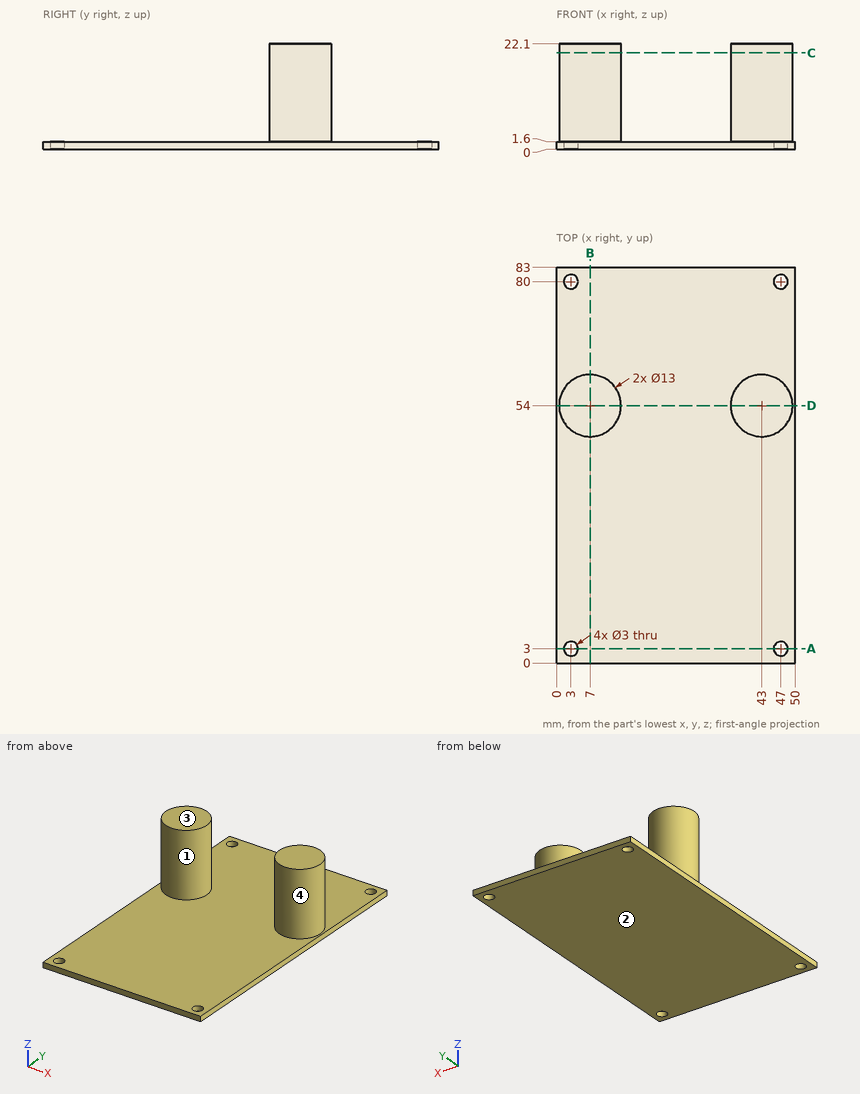
Design review of the part shown in the three views and the two pictorial views. Dimensions are in mm from the part's minimum x, y and z. A direction names the side the tool comes from. Round coordinates to 2 decimals unless told otherwise and drop trailing zeros. Loops run counter-clockwise (first coordinate to the right, second up) from the corner with the lowest first, then second, coordinate; pieces in that order, holes last.
1) Tool access review of the marked faces 3 and 4: name each direction out of +Z, -Z, +X, -X, +Y, -Y from which nothing blocks a thin tool from reaching the whole face with its end or side.
Values follow:
face 3: +Z, +X, -X, +Y, -Y
face 4: +Z
2) Clearance check with flat-ended pins moving along their axes: P1, Ø6, axis at y = 46, z = 8.5, coming from the +X side; P2, Ø8, axis at x = 29.5, y = 23.5, coming from the +Z side; P3, Ø1.8, axis at x = 3, y = 3, coming from the +Z side; P4, Ø8, axis at x = 35.5, z = 10, coming from the -Y side. State where each tip first meets the part, or that it passes through.
Values follow:
P1: stops at x = 47.15
P2: stops at z = 1.6
P3: passes through
P4: stops at y = 48.52
3) Consider section D-D on y = 54. State the section outline as (x, z) points, then the cut area to 3 significant figures.
Values follow:
outline: (0, 0) - (50, 0) - (50, 1.6) - (49.5, 1.6) - (49.5, 22.1) - (36.5, 22.1) - (36.5, 1.6) - (13.5, 1.6) - (13.5, 22.1) - (0.5, 22.1) - (0.5, 1.6) - (0, 1.6) - close
area: 613 mm2
4) Consider section B-B on x = 7. State the section outline as (y, z) points, then the cut area to 3 significant figures.
Values follow:
outline: (0, 0) - (83, 0) - (83, 1.6) - (60.5, 1.6) - (60.5, 22.1) - (47.5, 22.1) - (47.5, 1.6) - (0, 1.6) - close
area: 399 mm2
5) Wall thickness on line 1 along Y through (x, z) = (3, 0.4); line 2 along X through (y, z) = (80, 0.8); line 3 along Z through (x, y) = (14.5, 55.5): over which ranges is each line inside the solid? List them lowest first.
Values follow:
line 1: y = 0 to 1.5, 4.5 to 78.5, 81.5 to 83
line 2: x = 0 to 1.5, 4.5 to 45.5, 48.5 to 50
line 3: z = 0 to 1.6
6) Consider section A-A on y = 3. State the section outline as (x, z) points, then the cut area to 3 significant figures.
Values follow:
outline: (0, 0) - (1.5, 0) - (1.5, 1.6) - (0, 1.6) - close; (4.5, 0) - (45.5, 0) - (45.5, 1.6) - (4.5, 1.6) - close; (48.5, 0) - (50, 0) - (50, 1.6) - (48.5, 1.6) - close
area: 70.4 mm2
7) The part is to be moulded in two halves that separate along X. For the marked faces 1 and 2, say which applies: pulls with the +X half, pulls with the -X half, needs draft (parallel to the pull), parting line crosses it, or undercut.
Values follow:
face 1: undercut
face 2: needs draft
8) Consider section C-C on z = 20.25. State the section outline as (x, y) points.
Values follow:
outline: circle Ø13 at (7, 54); circle Ø13 at (43, 54)
